Input: dimensioned drawing with shaded views. Units: mm. Origin: part minimum x, y, z. A direction names the side the tool comes from. Give positions to 0.01 mm unless a question says otherwise; leave off trailing zeros. Write each loop counter-clockwise with the first axis right and the second up, starting at its lowest first coordinate (ties: lowest second). Pieces come first, ordered by that corner, then holes. Notation, with made-up numbers: M 73,40.25 L 80,40.25 A18 ccw 80,58.25 Z; hole C -3,66.25 d7. An arc over 180 degrees is marked long. Use CSV: the item, a comma, the result in double quotes. Start each with the question number.
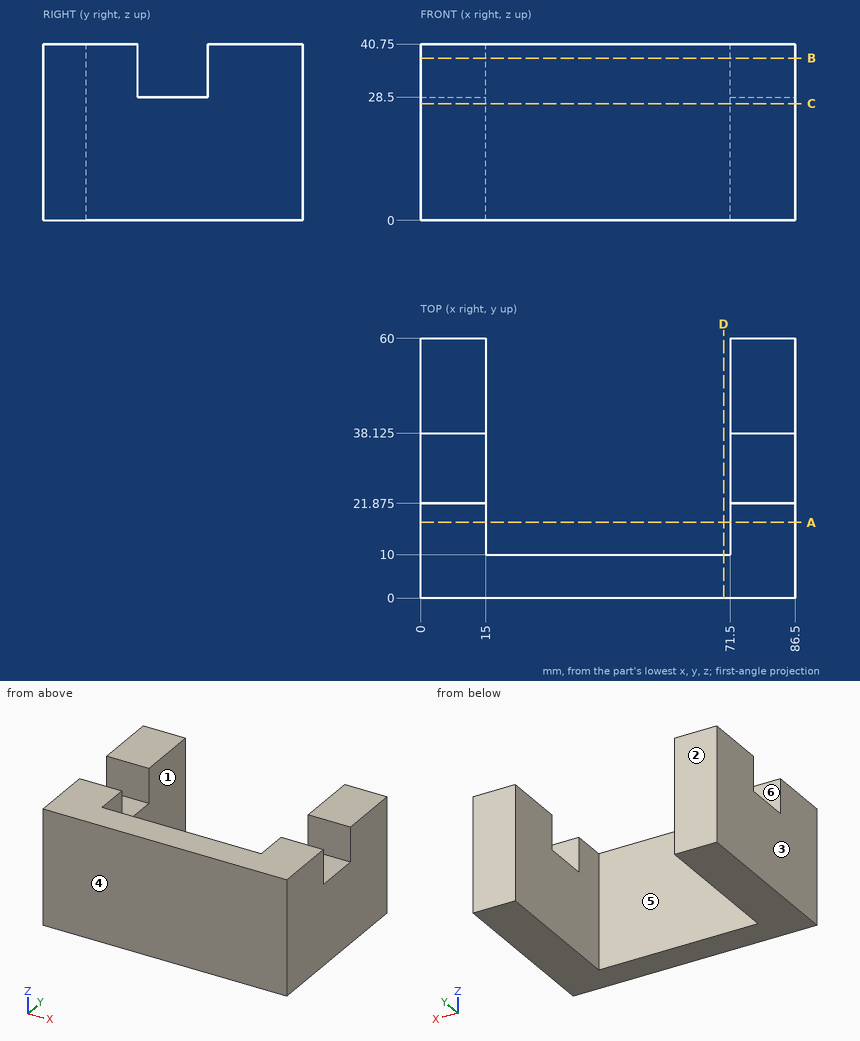
Item 1: Section B-B (z = 37.5). Return the cut outline in (x, y) (3 decimals).
Item 2: Material intervals for probe 1 along Y at (x, z) = (14.5, 35) (3 decimals); probe 2 along X at (y, z) = (14.5, 39); probe 3 along Z at (x, y) = (8, 25.5), sorted ascending.
Item 3: Set-up query: the marked faces 4, 5 and 6. Return all of +Z, -Z, +X, -X, +Y, -Y with unobstructed straight access to the full face (end or side cutting, diameter ignored); none if empty.
Item 4: Contact query for flat-ended pins moving along their axis: pin 1 Ø4 at (x, z) = (64, 36) entering from +Y; pin 2 Ø7.5 at (x, y) = (81.5, 33.5) entering from +Z. Output: stop coordinate, or through.
Item 5: Pull-direction query (X, two-part tool) for the marked faces 1, 2 and 3; classes: released by +X, released by -X, zero draft, split by the parting line, or undercut.
Item 6: Section D-D (x = 70). Return the cut outline in (y, z), plus the area to 4 significant figures.
Item 7: Section A-A (y = 17.5). Return the cut outline in (x, z).
Item 8: Section C-C (z = 27). Return the cut outline in (x, y).
Output values:
1,outline,"M 0,0 L 86.5,0 L 86.5,21.875 L 71.5,21.875 L 71.5,10 L 15,10 L 15,21.875 L 0,21.875 Z; M 0,38.125 L 15,38.125 L 15,60 L 0,60 Z; M 71.5,38.125 L 86.5,38.125 L 86.5,60 L 71.5,60 Z"
2,probe 1,"y = 0 to 21.875, 38.125 to 60"
2,probe 2,"x = 0 to 15, 71.5 to 86.5"
2,probe 3,"z = 0 to 28.5"
3,face 4,"+Z, -Z, +X, -X, -Y"
3,face 5,"+Z, -Z, +Y"
3,face 6,"+Z, +X, -X"
4,pin 1,"stops at y = 10"
4,pin 2,"stops at z = 28.5"
5,face 1,"undercut"
5,face 2,"zero draft"
5,face 3,"released by -X"
6,outline,"M 0,0 L 10,0 L 10,40.75 L 0,40.75 Z"
6,area,"407.5 mm2"
7,outline,"M 0,0 L 15,0 L 15,40.75 L 0,40.75 Z; M 71.5,0 L 86.5,0 L 86.5,40.75 L 71.5,40.75 Z"
8,outline,"M 0,0 L 86.5,0 L 86.5,60 L 71.5,60 L 71.5,10 L 15,10 L 15,60 L 0,60 Z"
